The listing builds one solid part. Answer for the finished solid, in the listing's coordinates (mm). Face numbers are marked on the shaded views. A direction names the side the tool comes from. Coordinates: 2 decimals unless noted, no trailing zeros. Write each loop counter-clockwise with the first axis right and the second up, starting at its lowest first coordinate (ties: lowest second). Pieces come first, ordered by that corner, then holes. Notation, with made-up numbers: M 71,70.25 L 102,70.25 A19 cw 102,74.25 Z; hole C 69,-36 d5. An arc over 180 degrees is marked long. Answer as CSV lines item,"result".
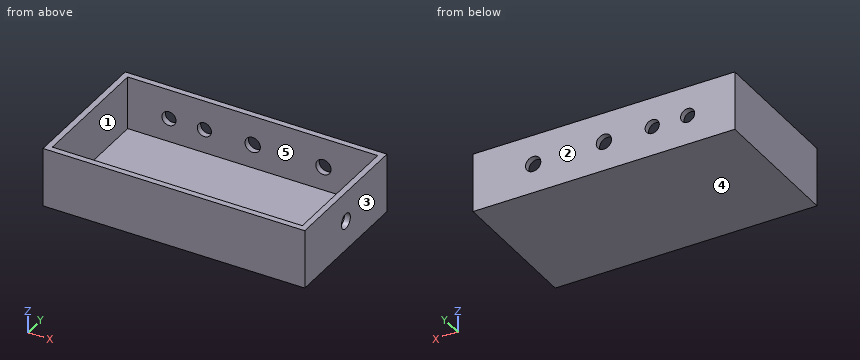
```python
from build123d import *

# Parameters (mm, degrees)
F0_W     = 111
F0_H     = 60
F1_DEPTH = 25
F2_T     = -2.5
F3_R     = 3.25
F4_DEPTH = 55.5
F5_R     = 3.25
F6_DEPTH = 30
F7_R     = 3
F8_DEPTH = 30


with BuildPart() as f1:
    # F0 (on Top) → F1 (new body)
    with BuildSketch(Plane.XY):
        Rectangle(F0_W, F0_H)
    extrude(amount=F1_DEPTH)

    # F2
    f2_openings = [f1.faces().sort_by_distance(p)[0] for p in [
        (0, 0, 25),
    ]]
    offset(amount=F2_T, openings=f2_openings)

    # F3 (on Right) → F4 (cut, through all)
    with BuildSketch(Plane.YZ):
        with Locations((0, 12.5)):
            Circle(F3_R)
    extrude(amount=F4_DEPTH, mode=Mode.SUBTRACT)

    # F5 (on Front) → F6 (cut, through all)
    with BuildSketch(Plane.XZ):
        with Locations((0, 12.5)):
            Circle(F5_R)
        with Locations((30, 12.5)):
            Circle(F5_R)
    extrude(amount=-F6_DEPTH, mode=Mode.SUBTRACT)

    # F7 (on Front) → F8 (cut, through all)
    with BuildSketch(Plane.XZ):
        with Locations((-35.5, 12.5)):
            Circle(F7_R)
        with Locations((-20.5, 12.5)):
            Circle(F7_R)
    extrude(amount=-F8_DEPTH, mode=Mode.SUBTRACT)


solid = f1.part
```
Q1. Flat-ended cylindrical pins translate along their axes: pin 1 Ø5.5 at (x, z) = (-35.5, 12.5) entering from +Y; pin 2 Ø16.5 at (x, y) = (-19, 3.5) entering from +Z. Find the tip coordinate at first contact, or state that the pin passes through.
Output:
pin 1,"y = -27.5"
pin 2,"z = 2.5"
Q2. Find section A-A (z = 12.5). Give the vertices of the cut face in (x, y), and give its area (3 significant figures).
Output:
outline,"M -55.5,-30 L 55.5,-30 L 55.5,-3.25 L 53,-3.25 L 53,-27.5 L -53,-27.5 L -53,27.5 L -38.5,27.5 L -38.5,30 L -55.5,30 Z; M -32.5,27.5 L -23.5,27.5 L -23.5,30 L -32.5,30 Z; M -17.5,27.5 L -3.25,27.5 L -3.25,30 L -17.5,30 Z; M 3.25,27.5 L 26.75,27.5 L 26.75,30 L 3.25,30 Z; M 33.25,27.5 L 53,27.5 L 53,3.25 L 55.5,3.25 L 55.5,30 L 33.25,30 Z"
area,"751 mm2"
Q3. The mould has two halves that part along Y. Classify the marked faces 1, 2 and 3: pulls with the +Y half, pulls with the -Y half, needs draft (parallel to the pull), parting line crosses it, or undercut.
Output:
face 1,"undercut"
face 2,"pulls with the +Y half"
face 3,"needs draft"
Q4. Find section C-C (y = 0). Give the vertices of the cut face in (x, z), and give its area (3 significant figures).
Output:
outline,"M -55.5,0 L 55.5,0 L 55.5,9.25 L 53,9.25 L 53,2.5 L -53,2.5 L -53,25 L -55.5,25 Z; M 53,15.75 L 55.5,15.75 L 55.5,25 L 53,25 Z"
area,"374 mm2"
Q5. Find section B-B (x = 0). Give the vertices of the cut face in (y, z), and give its area (3 significant figures).
Output:
outline,"M -30,0 L 30,0 L 30,9.25 L 27.5,9.25 L 27.5,2.5 L -27.5,2.5 L -27.5,25 L -30,25 Z; M 27.5,15.75 L 30,15.75 L 30,25 L 27.5,25 Z"
area,"246 mm2"
Q6. Straight lines are drawn through the part: line 1 (Y direction, x = -50, z = 10); line 2 (X direction, y = -9, z = 14.5); line 3 (Z direction, x = 30, y = 29.3). For each, find the intervals that lie inside material, in ascending order.
Output:
line 1,"-30 to -27.5, 27.5 to 30"
line 2,"-55.5 to -53, 53 to 55.5"
line 3,"0 to 9.25, 15.75 to 25"
Q7. For the marked faces 4 and 5, determine the directions among +Z, -Z, +X, -X, +Y, -Y from which every point of the face is accessible in a straight line to the end or side of a thin tool.
Output:
face 4,"-Z, +X, -X, +Y, -Y"
face 5,"+Z"
Q8. Find section D-D (y = -16.5). Give the vertices of the cut face in (x, z).
Output:
outline,"M -55.5,0 L 55.5,0 L 55.5,25 L 53,25 L 53,2.5 L -53,2.5 L -53,25 L -55.5,25 Z"
